Verification items for the finished model (mm, model axes). A direction names the side the tool comes from. Coordinates: 2 decimals unless noted, no trailing zeros. Write each loop counter-clockwise with the first axis right and the second up, starting at its lowest first coordinate (ties: lowest second). Pieces come first, ordered by that corner, then holes. Notation, with made-up numbers: (51.25, -39) -> (69.25, -39) arc R13 cw to (69.25, -21) -> close; hole circle Ø2 at (-10, 81). An arc over 180 degrees is marked (long way). Answer in a Markdown table with one row per item.
```python
from build123d import *

# Parameters (mm, degrees)
BOSS_EXTRUDE1_DEPTH = 3.175
BOSS_EXTRUDE2_DEPTH = 3.175
SKETCH3_W           = 6.236959702
SKETCH3_H           = 47.194711522
BOSS_EXTRUDE3_DEPTH = 3.175
SKETCH4_R           = 1.5
BOSS_EXTRUDE4_DEPTH = 3.175


with BuildPart() as part:
    # Sketch1 → Boss-Extrude1 (new body)
    with BuildSketch(Plane.XY):
        with BuildLine():
            Line((-17.114253333, -17.357583949), (-17.114253333, 17.357583949))
            ThreePointArc((-17.114253333, 17.357583949), (0, 24.432200125), (17.114253333, 17.357583949))
            Line((17.114253333, 17.357583949), (17.114253333, -17.357583949))
            ThreePointArc((17.114253333, -17.357583949), (0, -13.382802691), (-17.114253333, -17.357583949))
        make_face()
    extrude(amount=BOSS_EXTRUDE1_DEPTH)

    # Sketch2 → Boss-Extrude2 (add)
    with BuildSketch(Plane(origin=(0, 0, 0), x_dir=(-1, 0, 0), z_dir=(0, 0, -1))):
        with BuildLine():
            Line((-1.65128862, -13.417928303), (-1.65128862, 22.268343179))
            Line((-1.65128862, 22.268343179), (-1.65128862, 23.29835294))
            Line((-1.65128862, 23.29835294), (-2.853426735, 23.29835294))
            Line((-2.853426735, 23.29835294), (-2.853426735, -13.48778167))
            ThreePointArc((-2.853426735, -13.48778167), (-2.25262846, -13.448194961), (-1.65128862, -13.417928303))
        make_face()
        with BuildLine():
            Line((1.65128862, 23.29835294), (1.65128862, 22.268343179))
            Line((1.65128862, 22.268343179), (1.65128862, -13.417928303))
            ThreePointArc((1.65128862, -13.417928303), (2.25262846, -13.448194961), (2.853426735, -13.48778167))
            Line((2.853426735, -13.48778167), (2.853426735, 23.29835294))
            Line((2.853426735, 23.29835294), (1.65128862, 23.29835294))
        make_face()
    extrude(amount=BOSS_EXTRUDE2_DEPTH)

    # Sketch3 → Boss-Extrude3 (add)
    with BuildSketch(Plane.XY.offset(3.175)):
        with Locations((0, -23.258467244)):
            Rectangle(SKETCH3_W, SKETCH3_H)
    extrude(amount=-BOSS_EXTRUDE3_DEPTH)

    # Sketch4 → Boss-Extrude4 (add)
    with BuildSketch(Plane.XY.offset(3.175)):
        with Locations((0, -34.503683415)):
            Circle(SKETCH4_R)
    extrude(amount=BOSS_EXTRUDE4_DEPTH)


solid = part.part
```
1. Release check for a two-part mould opening along X. For faces 1 (the face through (0, 5, 3.175)), 2 (the face through (17.114, 0, 2)), 3 (the face through (-1.651, 5, -2)) record: released by +X, released by -X, zero draft, split by the parting line, or undercut.
Findings below:
| item | result |
|---|---|
| face 1 | zero draft |
| face 2 | released by +X |
| face 3 | undercut |
2. Sectioned sample at B-B, the plane y = 9. Record the cut outline in (x, z) (3 decimals), and give its area (3 significant figures).
Findings below:
| item | result |
|---|---|
| outline | (-17.114, 0) -> (-2.853, 0) -> (-2.853, -3.175) -> (-1.651, -3.175) -> (-1.651, 0) -> (1.651, 0) -> (1.651, -3.175) -> (2.853, -3.175) -> (2.853, 0) -> (17.114, 0) -> (17.114, 3.175) -> (-17.114, 3.175) -> close |
| area | 116 mm² |
3. Sectioned sample at D-D, the plane y = -28.5. Record the cut outline in (x, z) (3 decimals), and give its area (3 significant figures).
Findings below:
| item | result |
|---|---|
| outline | (-3.118, 0) -> (3.118, 0) -> (3.118, 3.175) -> (-3.118, 3.175) -> close |
| area | 19.8 mm² |
4. Go/stop test with flat-tipped pins: pin 1 (10.5 mm diameter, centred on x = 1, y = -4, fed in from +Z) (3 decimals); pin 2 (1 mm diameter, centred on y = -3, z = -2, fed in from -X); pin 3 (5 mm diameter, centred on x = 2.5, y = -23.5, fed in from -Z); pin 4 (1 mm diameter, centred on x = 4, y = -21.5, fed in from +Z). Record where each tip stops, or that it passes through.
Findings below:
| item | result |
|---|---|
| pin 1 | stops at z = 3.175 |
| pin 2 | stops at x = -2.85 |
| pin 3 | stops at z = 0 |
| pin 4 | passes through |
5. Access from +Z, -Z, +X, -X, +Y, -Y to the whole of each face (thin tool, end or side, straight path). Record for faces 4 (the face through (-2, 23.298, -2)), 5 (the face through (2.26, -13.45, -1.57)), 6 (the face through (1.651, 5, -2)), 7 (the face through (2.853, 5, -2)).
Findings below:
| item | result |
|---|---|
| face 4 | -Z, +X, -X, +Y |
| face 5 | -Z, -Y |
| face 6 | -Z, +Y, -Y |
| face 7 | -Z, +X, +Y, -Y |
6. Material ranges on probe 1 along X at (y, z) = (15.5, -1.25); probe 2 along Z at (x, y) = (5.5, 21) (3 decimals); probe 3 along X at (y, z) = (-34.5, 3.5), recorded low to high. Write a range as from..to.
Findings below:
| item | result |
|---|---|
| probe 1 | x = -2.85..-1.65, 1.65..2.85 |
| probe 2 | z = 0..3.175 |
| probe 3 | x = -1.5..1.5 |
7. Sectioned sample at A-A, the plane z = -1.75. Record the cut outline in (x, y).
Findings below:
| item | result |
|---|---|
| outline | (-2.85, -13.49) arc R38.83 cw to (-1.65, -13.42) -> (-1.65, 23.3) -> (-2.85, 23.3) -> close; (1.65, -13.42) arc R38.83 cw to (2.85, -13.49) -> (2.85, 23.3) -> (1.65, 23.3) -> close |
8. Sectioned sample at C-C, the plane x = 0. Record the cut outline in (y, z) (3 decimals), and give its area (3 significant figures).
Findings below:
| item | result |
|---|---|
| outline | (-46.856, 0) -> (24.432, 0) -> (24.432, 3.175) -> (-33.004, 3.175) -> (-33.004, 6.35) -> (-36.004, 6.35) -> (-36.004, 3.175) -> (-46.856, 3.175) -> close |
| area | 236 mm² |
